from build123d import *

# Parameters (mm, degrees)
F0_W     = 449.834
F0_H     = 697.781688
F1_DEPTH = 1630.68
F2_R     = 29.584786
F3_DEPTH = 167.64
F4_R     = 28.30083
F5_DEPTH = 167.64


with BuildPart() as f1:
    # F0 (on Front) → F1 (new body)
    with BuildSketch(Plane.XZ):
        with Locations((-1.818407, 114.559772)):
            Rectangle(F0_W, F0_H)
    extrude(amount=F1_DEPTH)

    # F2 (on face) → F3 (join)
    with BuildSketch(Plane.XZ.offset(1630.68)):
        Circle(F2_R)
    extrude(amount=F3_DEPTH)

    # F4 (on face) → F5 (join)
    with BuildSketch(Plane(origin=(0, 0, 0), x_dir=(-1, 0, 0), z_dir=(0, 1, 0))):
        Circle(F4_R)
    extrude(amount=F5_DEPTH)


solid = f1.part
Geometry check sheet. Reference: the model listing, model coordinates, mm. A direction names the side the tool comes from. Coordinates: 2 decimals unless noted, no trailing zeros. Order: outer loops, then holes, each group sorted by start corner. A loop starts at its lowest first (then second) coordinate and runs counter-clockwise, first axis right, second up. Notation, with made-up numbers: (71, 45.25) -> (113, 45.25) arc R24 cw to (113, 65.25) -> close; hole circle Ø10 at (69.5, 67.5). An arc over 180 degrees is marked (long way). Use a Markdown table: item, result. Add a question column.
1. Set-up check for faces 1 (the face through (27.33, -1713.33, -11.33)), 2 (the face through (0, 167.64, 0)), 3 (the face through (6.135, 82.647, -27.628)): record each of +Z, -Z, +X, -X, +Y, -Y from which the full face is reachable in a straight line by a thin tool's end or side.
2. Cross-section at A-A (z = 0). Enter the section's corners in (x, y), and give its area (3 significant figures).
3. Cross-section at B-B (x = 0). Enter the section's corners in (y, z), and give its area (3 significant figures).
4. Go/stop test with flat-tipped pins: pin 1 Ø8 at (x, z) = (-169, 365.5) entering from +Y; pin 2 Ø4 at (x, z) = (-88, 52) entering from -Y. Record where each tip stops, or that it passes through.
5. Material ranges on L1, parallel to Y at x = 23.5, z = -182, recorded low to high.
Filled sheet:
| question | item | result |
|---|---|---|
| 1 | face 1 | -Y |
| 1 | face 2 | +Z, -Z, +X, -X, +Y |
| 1 | face 3 | +Y |
| 2 | outline | (-226.74, -1630.68) -> (-29.58, -1630.68) -> (-29.58, -1798.32) -> (29.58, -1798.32) -> (29.58, -1630.68) -> (223.1, -1630.68) -> (223.1, 0) -> (28.3, 0) -> (28.3, 167.64) -> (-28.3, 167.64) -> (-28.3, 0) -> (-226.74, 0) -> close |
| 2 | area | 753,000 mm2 |
| 3 | outline | (-1798.32, -29.58) -> (-1630.68, -29.58) -> (-1630.68, -234.33) -> (0, -234.33) -> (0, -28.3) -> (167.64, -28.3) -> (167.64, 28.3) -> (0, 28.3) -> (0, 463.45) -> (-1630.68, 463.45) -> (-1630.68, 29.58) -> (-1798.32, 29.58) -> close |
| 3 | area | 1,160,000 mm2 |
| 4 | pin 1 | y = 0 |
| 4 | pin 2 | y = -1630.68 |
| 5 | L1 | -1630.68 to 0 |
